Work out the finished part from the listing and answer in its coordinate system (mm). Face numbers are marked on the shaded views. Give positions to 0.01 mm unless a question says otherwise; leave off trailing zeros. Loops run counter-clockwise (first coordinate to the right, second up) from the corner with the lowest first, then second, coordinate; pieces in that order, holes last. Notation, with made-up numbers: (12.5, -8) - (47.5, -8) arc R15 cw to (47.5, 12) - close; hole circle Ø11 at (-30, -25). An arc over 180 degrees is marked (long way). One line per item, written item: value.
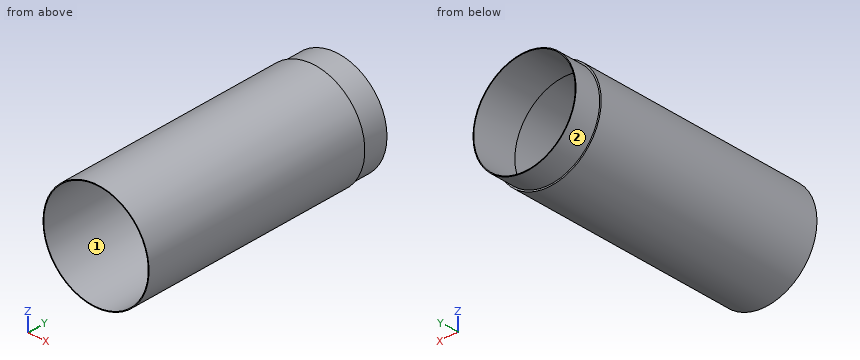
Autodesk Inventor part; units mm, degrees
ref_plane "Work Plane2" through (35, 0, 0) normal (1, 0, 0) x (0, 1, 0)
ref_plane "Work Plane4" through (34, 0, 0) normal (1, 0, 0) x (0, 1, 0)
ref_plane "XZ Plane" through (0, 0, 0) normal (0, 1, 0) x (-1, 0, 0)
sketch "Sketch1" plane through (0, 0, 0) normal (0, 1, 0) x (-1, 0, 0)
  circle A0 centre (0, 0) radius 35
  circle A1 centre (0, 0) radius 34.5
  dimension "d0" = 70
  dimension "d1" = 69
extrude "Extrusion1" add sketch "Sketch1" along normal blind 155
ref_plane "Work Plane2" through (35, 0, 0) normal (1, 0, 0) x (0, 1, 0)
sketch "Sketch5" plane through (0, 155, 0) normal (0, 1, 0) x (1, 0, 0)
  circle A0 centre (0, 0) radius 34
  circle A1 centre (0, 0) radius 33.5
  dimension "d44" = 68
  dimension "d45" = 67
extrude "Extrusion3" add sketch "Sketch5" along normal blind 17
sketch "Sketch6" plane through (0, 155, 0) normal (0, -1, 0) x (1, 0, 0)
  circle A0 centre (0, 0) radius 33.5
  circle A1 centre (0, 0) radius 34.5
  circle A2 centre (0, 0) radius 35
extrude "Extrusion4" add sketch "Sketch6" along normal blind 12.5 contours A1
ref_plane "Work Plane4" through (34, 0, 0) normal (1, 0, 0) x (0, 1, 0)
properties part number "Engine skin lower" material "Plastic, Opaque White"
1. Find the intervals of material crossed by line 1 along Z through (x, y) = (0, 87); line 2 along X through (y, z) = (164.25, 0); line 3 along Z through (x, y) = (-17, 81), in increasing order.
Output:
line 1: z = -35 to -34.5, 34.5 to 35
line 2: x = -34 to -33.5, 33.5 to 34
line 3: z = -30.59 to -30.02, 30.02 to 30.59
2. Flat-ended cylindrical pins translate along their axes: pin 1 Ø4 at (y, z) = (19, -8) entering from +X; pin 2 Ø12 at (x, z) = (-2.5, -27.5) entering from -Y; pin 3 Ø3 at (y, z) = (132.5, -19.5) entering from +X. Find the tip coordinate at first contact, or state that the pin passes through.
Output:
pin 1: stops at x = 34.48
pin 2: stops at y = 142.5
pin 3: stops at x = 30.02
3. The mould has two halves that part along Z. Classify the marked faces 1 and 2: released by +Z, released by -Z, zero draft, split by the parting line, or undercut.
Output:
face 1: undercut
face 2: split by the parting line
4. Section A-A (x = 0) is taken. Write down the section's boundary in (y, z), and give its area (3 significant figures).
Output:
outline: (0, -35) - (155, -35) - (155, -34) - (172, -34) - (172, -33.5) - (142.5, -33.5) - (142.5, -34.5) - (0, -34.5) - close; (0, 34.5) - (142.5, 34.5) - (142.5, 33.5) - (172, 33.5) - (172, 34) - (155, 34) - (155, 35) - (0, 35) - close
area: 197 mm²
5. Section C-C (y = 26.5) is taken. Write down the section's boundary in (x, z).
Output:
outline: circle Ø70 at (0, 0); hole circle Ø69 at (0, 0)
6. Section B-B (z = 0) is taken. Write down the section's boundary in (x, y).
Output:
outline: (-35, 0) - (-34.5, 0) - (-34.5, 142.5) - (-33.5, 142.5) - (-33.5, 172) - (-34, 172) - (-34, 155) - (-35, 155) - close; (33.5, 142.5) - (34.5, 142.5) - (34.5, 0) - (35, 0) - (35, 155) - (34, 155) - (34, 172) - (33.5, 172) - close
